from build123d import *

# Parameters (mm, degrees)
BOSS_EXTRUDE4_DEPTH = 965.2
SKETCH61_R          = 50.8
SKETCH61_R_2        = 25.4
BOSS_EXTRUDE5_DEPTH = 50.8
BOSS_EXTRUDE6_DEPTH = 50.8


with BuildPart() as part:
    # Sketch1 → Boss-Extrude4 (new body)
    with BuildSketch(Plane.XY):
        Polygon((-203.2, 25.4), (-254, -25.4), (-236.039487758, -25.4), (-223.339487758, -12.7), (-197.939487758, 12.7), (-185.239487758, 25.4), align=None)
        Polygon((203.2, 25.4), (-185.239487758, 25.4), (-197.939487758, 12.7), (197.939487758, 12.7), (223.339487758, -12.7), (236.039487758, -25.4), (254, -25.4), align=None)
    extrude(amount=BOSS_EXTRUDE4_DEPTH)


with BuildPart() as part_1:
    # Body-Move/Copy1: moved
    add(part.part.moved(Location((0, 0, -482.6))))

    # Sketch61 → Boss-Extrude5 (add)
    # profile 1 of 4: a face of its own
    with BuildSketch(Plane.XZ.offset(-12.7)):
        with Locations((-145.808181247, 254)):
            Circle(SKETCH61_R)
        with Locations(Location((-145.808181247, 254, 0), (0, 0, 180))):
            Circle(SKETCH61_R_2, mode=Mode.SUBTRACT)
    # profile 2 of 4: a face of its own
    with BuildSketch(Plane.XZ.offset(-12.7)):
        with Locations(Location((145.808181247, 254, 0), (0, 0, 180))):
            Circle(SKETCH61_R)
        with Locations((145.808181247, 254)):
            Circle(SKETCH61_R_2, mode=Mode.SUBTRACT)
    # profile 3 of 4: a face of its own
    with BuildSketch(Plane.XZ.offset(-12.7)):
        with Locations((145.808181247, -254)):
            Circle(SKETCH61_R)
        with Locations(Location((145.808181247, -254, 0), (0, 0, 180))):
            Circle(SKETCH61_R_2, mode=Mode.SUBTRACT)
    # profile 4 of 4: a face of its own
    with BuildSketch(Plane.XZ.offset(-12.7)):
        with Locations(Location((-145.808181247, -254, 0), (0, 0, 180))):
            Circle(SKETCH61_R)
        with Locations((-145.808181247, -254)):
            Circle(SKETCH61_R_2, mode=Mode.SUBTRACT)
    extrude(amount=BOSS_EXTRUDE5_DEPTH)

    # Sketch62 → Boss-Extrude6 (add)
    with BuildSketch(Plane(origin=(0, 25.4, 0), x_dir=(1, 0, 0), z_dir=(0, 1, 0))):
        Polygon((0, -92.772173632), (65.599833081, -65.599833081), (92.772173632, 0), (65.599833081, 65.599833081), (0, 92.772173632), (-65.599833081, 65.599833081), (-92.772173632, 0), (-65.599833081, -65.599833081), align=None)
    extrude(amount=BOSS_EXTRUDE6_DEPTH)


solid = part_1.part
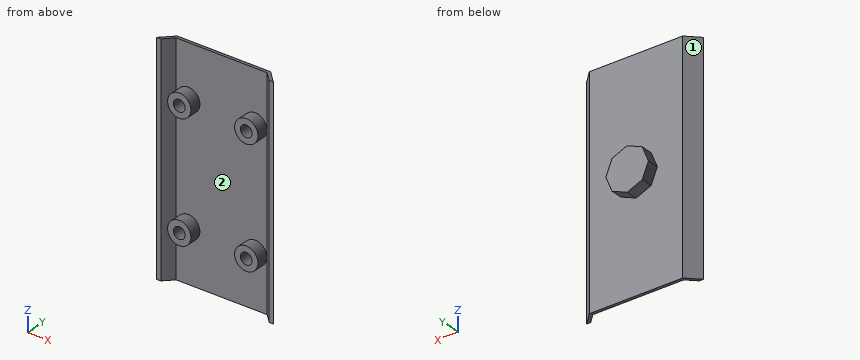
Work out the finished part from the listing and answer in its coordinate system (mm). Face numbers are marked on the shaded views. Round coordinates to 2 decimals unless told otherwise and drop trailing zeros. Write each loop counter-clockwise with the first axis right and the second up, starting at its lowest first coordinate (ties: lowest second). Pieces come first, ordered by that corner, then holes. Notation, with made-up numbers: (-28, 32.5) -> (-7, 32.5) arc R7 cw to (-7, 45.5) -> close; hole circle Ø11 at (5.25, 7.5). An arc over 180 degrees is marked (long way). Write each question's results on one line, items separated by ' | '.
Item 1: Find the intervals of material crossed by line 1 along Y through (x, z) = (99.5, -364); line 2 along Y through (x, z) = (169, 281.5); line 3 along X through (y, z) = (-10.5, -225), in increasing order. Write a range as [from, to].
Result set:
line 1: [12.7, 25.4] | line 2: [-38.1, 25.4] | line 3: [-239.1, -221.14], [-187.52, -104.1], [104.1, 187.52], [221.14, 239.1]
Item 2: The mould has two halves that part along Z. Classify the marked faces 1 and 2: +Z half, -Z half, draft (parallel to the pull), parting line (faces both ways), or undercut.
Result set:
face 1: draft | face 2: undercut
Item 3: A cutting plane is placed at C-C, the plane x = 137. Determine the outline of the cut face in (y, z).
Result set:
outline: (-38.1, -304.03) -> (12.7, -304.03) -> (12.7, -482.6) -> (25.4, -482.6) -> (25.4, 482.6) -> (12.7, 482.6) -> (12.7, 304.03) -> (-38.1, 304.03) -> (-38.1, 277.82) -> (12.7, 277.82) -> (12.7, 230.18) -> (-38.1, 230.18) -> (-38.1, 203.97) -> (12.7, 203.97) -> (12.7, -203.97) -> (-38.1, -203.97) -> (-38.1, -230.18) -> (12.7, -230.18) -> (12.7, -277.82) -> (-38.1, -277.82) -> close
Item 4: A cutting plane is placed at B-B, the plane z = 342.5. Determine the outline of the cut face in (x, y).
Result set:
outline: (-254, -25.4) -> (-236.04, -25.4) -> (-197.94, 12.7) -> (197.94, 12.7) -> (236.04, -25.4) -> (254, -25.4) -> (203.2, 25.4) -> (-203.2, 25.4) -> close
Item 5: A cutting plane is placed at A-A, the plane y = -8. Count the separate pieces of the cut face and the enclosed holes in it, plus the area to 3 significant figures.
Result set:
separate pieces: 6 | enclosed holes: 4 | area: 59,000 mm^2
Item 6: Flat-ended cylindrical pins translate along their axes: P1, Ø5.5, axis at x = -245, z = -241.5, coming from the -Y side; P2, Ø8, axis at x = -200.5, z = -70, coming from the -Y side; P3, Ø5, axis at x = -108.5, z = 2.5, coming from the -Y side. Find the tip coordinate at first contact, or state that the pin passes through.
Result set:
P1: y = -25.4 | P2: y = 6.14 | P3: y = 12.7
Item 7: A cutting plane is placed at D-D, the plane z = -11.5. Determine the outline of the cut face in (x, y).
Result set:
outline: (-254, -25.4) -> (-236.04, -25.4) -> (-197.94, 12.7) -> (197.94, 12.7) -> (236.04, -25.4) -> (254, -25.4) -> (203.2, 25.4) -> (88.01, 25.4) -> (88.01, 76.2) -> (-88.01, 76.2) -> (-88.01, 25.4) -> (-203.2, 25.4) -> close
